```python
from build123d import *

# Parameters (mm, degrees)
F2_R = 5
F3_T = -10


with BuildPart() as f1:
    # F0 (on Front) → F1 (revolve)
    with BuildSketch(Plane.XZ):
        with BuildLine():
            Line((0, 0), (0, -200))
            ThreePointArc((0, -200), (44.72135955, -194.9358868962), (87.1779788708, -180))
            ThreePointArc((87.1779788708, -180), (169.4632641226, -106.2177109192), (200, 0))
            Line((200, 0), (0, 0))
        make_face()
        with BuildLine():
            ThreePointArc((87.1779788708, -180), (44.72135955, -194.9358868962), (0, -200))
            Line((0, -200), (87.1779788708, -200))
            Line((87.1779788708, -200), (87.1779788708, -180))
        make_face()
    revolve(axis=Axis((0, 0, -100), (0, 0, 1)))

    # F2
    f2_edges = [f1.edges().sort_by_distance(p)[0] for p in [
        (-87.177979, 0, -180),
    ]]
    fillet(f2_edges, radius=F2_R)

    # F3
    f3_openings = [f1.faces().sort_by_distance(p)[0] for p in [
        (0, 0, 0),
    ]]
    offset(amount=F3_T, openings=f3_openings)


with BuildPart() as f5:
    # F4 (on face) → F5 (revolve)
    with BuildSketch(Plane.XZ):
        with BuildLine():
            Line((190, 0), (189.8106289646, -8.4808685904))
            ThreePointArc((189.8106289646, -8.4808685904), (189.9526513414, -4.2414912895), (190, 0))
        make_face()
    revolve(axis=Axis((0, 0, -100), (0, 0, 1)))


with BuildPart() as f5b:
    # F4 (on face) → F5, piece 2 (revolve)
    with BuildSketch(Plane.XZ):
        with BuildLine():
            ThreePointArc((189.8106289646, -8.4808685904), (188.6642077169, -22.4903696405), (186.4852005998, -36.3767777193))
            Line((186.4852005998, -36.3767777193), (189.215494745, -35.1335987777))
            Line((189.215494745, -35.1335987777), (189.8106289646, -8.4808685904))
        make_face()
    revolve(axis=Axis((0, 0, -100), (0, 0, 1)))


with BuildPart() as f5c:
    # F4 (on face) → F5, piece 3 (revolve)
    with BuildSketch(Plane.XZ):
        with BuildLine():
            Line((186.4852005998, -36.3767777193), (186.0620361102, -38.4827067462))
            ThreePointArc((186.0620361102, -38.4827067462), (186.2765944217, -37.4303402423), (186.4852005998, -36.3767777193))
        make_face()
    revolve(axis=Axis((0, 0, -100), (0, 0, 1)))


with BuildPart() as f5d:
    # F4 (on face) → F5, piece 4 (revolve)
    with BuildSketch(Plane.XZ):
        with BuildLine():
            ThreePointArc((186.0620361102, -38.4827067462), (182.3054866364, -53.5229814405), (177.3353102124, -68.2069479736))
            Line((177.3353102124, -68.2069479736), (180.2400008123, -67.4567663163))
            Line((180.2400008123, -67.4567663163), (186.0620361102, -38.4827067462))
        make_face()
    revolve(axis=Axis((0, 0, -100), (0, 0, 1)))


with BuildPart() as f5e:
    # F4 (on face) → F5, piece 5 (revolve)
    with BuildSketch(Plane.XZ):
        with BuildLine():
            Line((177.3353102124, -68.2069479736), (176.5528838044, -70.207401464))
            ThreePointArc((176.5528838044, -70.207401464), (176.9469240187, -69.2082804319), (177.3353102124, -68.2069479736))
        make_face()
    revolve(axis=Axis((0, 0, -100), (0, 0, 1)))


with BuildPart() as f5f:
    # F4 (on face) → F5, piece 6 (revolve)
    with BuildSketch(Plane.XZ):
        with BuildLine():
            ThreePointArc((176.5528838044, -70.207401464), (170.2416884657, -84.36686262), (162.7971761601, -97.9646846281))
            Line((162.7971761601, -97.9646846281), (165.7880056607, -97.7302941451))
            Line((165.7880056607, -97.7302941451), (176.5528838044, -70.207401464))
        make_face()
    revolve(axis=Axis((0, 0, -100), (0, 0, 1)))


with BuildPart() as f5g:
    # F4 (on face) → F5, piece 7 (revolve)
    with BuildSketch(Plane.XZ):
        with BuildLine():
            Line((162.7971761601, -97.9646846281), (161.6792614643, -99.7988798151))
            ThreePointArc((161.6792614643, -99.7988798151), (162.2408108688, -98.8833620415), (162.7971761601, -97.9646846281))
        make_face()
    revolve(axis=Axis((0, 0, -100), (0, 0, 1)))


with BuildPart() as f5h:
    # F4 (on face) → F5, piece 8 (revolve)
    with BuildSketch(Plane.XZ):
        with BuildLine():
            ThreePointArc((161.6792614643, -99.7988798151), (153.0051827375, -112.6472993705), (143.3125322896, -124.7458139127))
            Line((143.3125322896, -124.7458139127), (146.2986258499, -125.0343364403))
            Line((146.2986258499, -125.0343364403), (161.6792614643, -99.7988798151))
        make_face()
    revolve(axis=Axis((0, 0, -100), (0, 0, 1)))


with BuildPart() as f5i:
    # F4 (on face) → F5, piece 9 (revolve)
    with BuildSketch(Plane.XZ):
        with BuildLine():
            Line((143.3125322896, -124.7458139127), (141.8930965783, -126.3580197037))
            ThreePointArc((141.8930965783, -126.3580197037), (142.6050927785, -125.553922733), (143.3125322896, -124.7458139127))
        make_face()
    revolve(axis=Axis((0, 0, -100), (0, 0, 1)))


with BuildPart() as f5j:
    # F4 (on face) → F5, piece 10 (revolve)
    with BuildSketch(Plane.XZ):
        with BuildLine():
            ThreePointArc((141.8930965783, -126.3580197037), (131.1196919561, -137.5050049319), (119.4734096451, -147.736604766))
            Line((119.4734096451, -147.736604766), (122.3640363234, -148.5392736932))
            Line((122.3640363234, -148.5392736932), (141.8930965783, -126.3580197037))
        make_face()
    revolve(axis=Axis((0, 0, -100), (0, 0, 1)))


with BuildPart() as f5k:
    # F4 (on face) → F5, piece 11 (revolve)
    with BuildSketch(Plane.XZ):
        with BuildLine():
            Line((119.4734096451, -147.736604766), (117.795581754, -149.0778351038))
            ThreePointArc((117.795581754, -149.0778351038), (118.6363911057, -148.4095910156), (119.4734096451, -147.736604766))
        make_face()
    revolve(axis=Axis((0, 0, -100), (0, 0, 1)))


with BuildPart() as f5l:
    # F4 (on face) → F5, piece 12 (revolve)
    with BuildSketch(Plane.XZ):
        with BuildLine():
            Line((92.004147905, -166.2384936417), (94.7114774724, -167.5309202794))
            Line((94.7114774724, -167.5309202794), (117.795581754, -149.0778351038))
            ThreePointArc((117.795581754, -149.0778351038), (105.2501956844, -158.1846904994), (92.004147905, -166.2384936417))
        make_face()
    revolve(axis=Axis((0, 0, -100), (0, 0, 1)))


with BuildPart() as f1_1:
    add(f1.part)

    # F6: cut F5, F5b, F5c, F5d, F5e, F5f, F5g, F5h, F5i, F5j, F5k, F5l
    add(f5.part, mode=Mode.SUBTRACT)
    add(f5b.part, mode=Mode.SUBTRACT)
    add(f5c.part, mode=Mode.SUBTRACT)
    add(f5d.part, mode=Mode.SUBTRACT)
    add(f5e.part, mode=Mode.SUBTRACT)
    add(f5f.part, mode=Mode.SUBTRACT)
    add(f5g.part, mode=Mode.SUBTRACT)
    add(f5h.part, mode=Mode.SUBTRACT)
    add(f5i.part, mode=Mode.SUBTRACT)
    add(f5j.part, mode=Mode.SUBTRACT)
    add(f5k.part, mode=Mode.SUBTRACT)
    add(f5l.part, mode=Mode.SUBTRACT)


solid = f1_1.part
```
Check sheet for the modelled part. Datum: model origin and axes. Units: mm. A direction names the side the tool comes from. Give positions to 0.01 mm unless a question says otherwise; leave off trailing zeros. Loops run counter-clockwise (first coordinate to the right, second up) from the corner with the lowest first, then second, coordinate; pieces in that order, holes last. Notation, with made-up numbers: M 39.25,64 L 55.25,64 A15 ccw 55.25,91 Z; hole C 43.25,-30 d6. An arc over 180 degrees is marked long. Answer as CSV lines item,"result".
Item 1: Depth check by flat-ended pin: pin 1 Ø2 at (x, z) = (-36, -143.5) entering from -Y; pin 2 Ø10 at (x, z) = (-1, -174.5) entering from +Y; pin 3 Ø3 at (y, z) = (5.5, -157.5) entering from +X. Enter the tip coordinate at first touch or a pass-through.
Reply:
pin 1,"y = -135.67"
pin 2,"y = 106.15"
pin 3,"x = 125.04"
Item 2: Sectioned sample at B-B, the plane z = -134. Enter the section's corners in (x, y), then the cut area to 3 significant figures.
Reply:
outline,"C 0,0 d296.94; hole C 0,0 d270.33"
area,"11,900 mm^2"
Item 3: Sectioned sample at A-A, the plane z = -83. Enter the section's corners in (x, y).
Reply:
outline,"C 0,0 d363.93; hole C 0,0 d343.1"
Item 4: Scan lines: L1, parallel to X at y = 0, z = -186.5; L2, parallel to X at y = 44, z = -97.5. Record each from-to range of solid material in increasing order.
Reply:
L1,"-87.18 to -77.18, 77.18 to 87.18"
L2,"-168.99 to -159.94, 159.94 to 168.99"
Item 5: Set-up check for faces 1 (the face through (-18.898, -85.105, -191.435)), 2 (the face through (177, -73, 0)), 3 (the face through (73.614, 23.182, -186.505)): record each of +Z, -Z, +X, -X, +Y, -Y from which the full face is reachable in a straight line by a thin tool's end or side.
Reply:
face 1,"-Z"
face 2,"+Z, +X, -X, +Y, -Y"
face 3,"+Z"
